Model file for the job. Use its own axes, mm. A direction names the side the tool comes from. Coordinates: 2 decimals unless noted, no trailing zeros. Loops run counter-clockwise (first coordinate to the right, second up) from the corner with the lowest first, then second, coordinate; pieces in that order, holes last. Notation, with made-up numbers: M 6.5,16.5 L 32.5,16.5 A30 cw 32.5,45.5 Z; hole C 26.25,41.25 d2. An arc over 180 degrees is marked long. One line per question, with ' | ' between items. Start each with the question number.
```python
from build123d import *

# Parameters (mm, degrees)
F0_R      = 16.5
F1_DEPTH  = 5
F2_R      = 16.5
F2_R_2    = 15
F3_DEPTH  = 30
F4_R      = 12.2
F4_R_2    = 9.7
F5_DEPTH  = 27
F6_R      = 10.5
F7_DEPTH  = 30
F8_R      = 9.5
F8_R_2    = 8
F8_R_3    = 6.5
F9_DEPTH  = 30
F10_DEPTH = 30
F11_SIZE2 = 0.610917
F11_SIZE  = 34.99999


# Not quite as in the source:
# - a fillet or chamfer is up to 0.001 mm smaller than in the source, because OpenCascade refuses the exact size


with BuildPart() as f1:
    # F0 (on Top) → F1 (new body)
    with BuildSketch(Plane.XY):
        Circle(F0_R)
    extrude(amount=F1_DEPTH)

    # F2 (on face) → F3 (join)
    with BuildSketch(Plane.XY.offset(5)):
        Circle(F2_R)
        Circle(F2_R_2, mode=Mode.SUBTRACT)
    extrude(amount=F3_DEPTH)

    # F4 (on face) → F5 (join)
    with BuildSketch(Plane.XY.offset(5)):
        Circle(F4_R)
        Circle(F4_R_2, mode=Mode.SUBTRACT)
    extrude(amount=F5_DEPTH)

    # F6 (on face) → F7 (join)
    with BuildSketch(Plane(origin=(0, 0, 0), x_dir=(1, 0, 0), z_dir=(0, 0, -1))):
        Circle(F6_R)
    extrude(amount=F7_DEPTH)

    # F8 (on face) → F9 (cut)
    with BuildSketch(Plane(origin=(0, 0, -30), x_dir=(1, 0, 0), z_dir=(0, 0, -1))):
        Circle(F8_R)
        Circle(F8_R_2, mode=Mode.SUBTRACT)
        Circle(F8_R_3)
    extrude(amount=-F9_DEPTH, mode=Mode.SUBTRACT)

    # F10 (cut): a face of the model
    f10_faces = [f1.faces().sort_by_distance(p)[0] for p in [
        (0, 0, 0),
    ]]
    extrude(f10_faces, amount=-F10_DEPTH, mode=Mode.SUBTRACT)

    # F11 (size 35 and 0.6109272725 in the source; OpenCascade refuses exactly that, so slightly less here)
    f11_edges = [f1.edges().sort_by_distance(p)[0] for p in [
        (-6.5, 0, 5),
    ]]
    f11_side = f1.faces().sort_by_distance((-6.5, 0, -12.5))[0]
    chamfer(f11_edges, length=F11_SIZE, length2=F11_SIZE2, reference=f11_side)


solid = f1.part
```
(1) Two-plate mould, pull along X, no slides. Class faces 1 (the face through (-12.19, 0.54, 18.31)), 2 (the face through (-5, 9, -30)), 3 (the face through (10, -3.2, -14.8)): pulls with the +X half, pulls with the -X half, needs draft (parallel to the pull), parting line crosses it, or undercut.
(2) Band-saw the part on C-C on x = 13.5. Write the cut outline in (y, z).
(3) Drill centre lines: line 1 (Y direction, x = 0, z = 11.75); line 2 (Y direction, x = 8.5, z = 10); line 3 (X direction, y = -9, z = 8). Where is each one in solid material? Low to high. Write a range as [from, to].
(4) Band-saw the part on A-A on z = 31. Write the cut outline in (x, y).
(5) Pin check, flat tips, straight feed: P1, Ø11.5, axis at x = 0, y = 0, coming from the +Z side; P2, Ø1, axis at x = 6.5, y = -7.5, coming from the +Z side; P3, Ø8, axis at x = 12.5, z = 24, coming from the +Y side; P4, Ø10, axis at y = 11.5, z = 1, coming from the -X side. Stop position of each tip, or through.
(6) Band-saw the part on D-D on z = 3. Write the cut outline in (x, y), then the cut area to 3 significant figures.
(7) 3-axis set-ups, long thin cutter, end or side, ignore diameter. For faces 4 (the face through (4, -15, 35)), 5 (the face through (9.252, 2.914, 18.311)), 6 (the face through (0, -11, 0)): which of +Z, -Z, +X, -X, +Y, -Y reach the whole face in a straight line?
(8) Band-saw the part on B-B on y = 11.5. Write the cut outline in (x, z).
Computed values:
1) face 1: undercut | face 2: needs draft | face 3: parting line crosses it
2) outline: M -9.49,0 L 9.49,0 L 9.49,35 L 6.54,35 L 6.54,5 L -6.54,5 L -6.54,35 L -9.49,35 Z
3) line 1: [-16.5, -15], [-12.2, -9.7], [9.7, 12.2], [15, 16.5] | line 2: [-14.14, -12.36], [-8.75, -4.67], [4.67, 8.75], [12.36, 14.14] | line 3: [-13.83, -12], [-8.24, -3.62], [3.62, 8.24], [12, 13.83]
4) outline: C 0,0 d33; C 0,0 d24.4; hole C 0,0 d30; hole C 0,0 d19.4
5) P1: through | P2: z = 32 | P3: y = 14.14 | P4: x = -15.17
6) outline: C 0,0 d33; hole C 0,0 d14.15 | area: 698 mm^2
7) face 4: +Z, +X, -X, +Y, -Y | face 5: +Z | face 6: -Z
8) outline: M -11.83,0 L 11.83,0 L 11.83,35 L 9.63,35 L 9.63,5 L 4.07,5 L 4.07,32 L -4.07,32 L -4.07,5 L -9.63,5 L -9.63,35 L -11.83,35 Z
